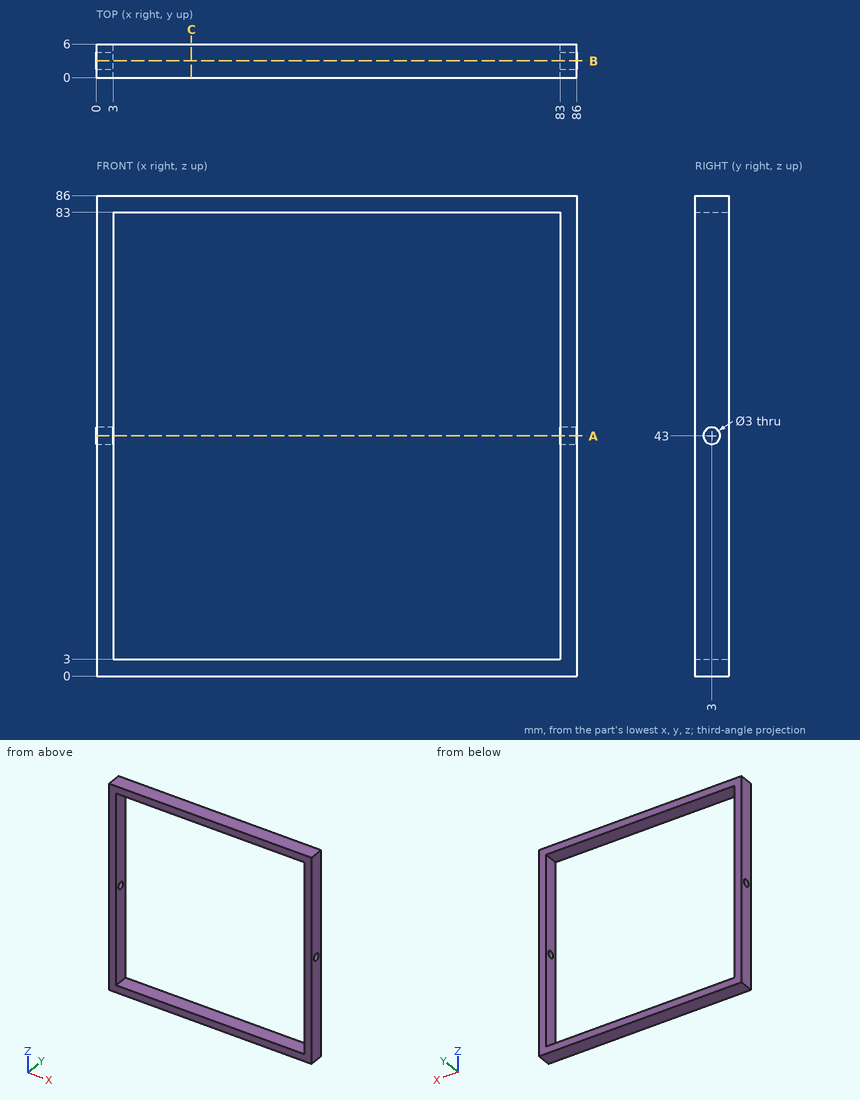
Can you work these out from the drawing? Everything is in mm from the part's minimum corner. Coordinates: 2 decimals unless noted, no trailing zeros. Loops run counter-clockwise (first coordinate to the right, second up) from the corner with the lowest first, then second, coordinate; pieces in that order, holes last. Notation, with made-up numbers: (54.25, 7) - (83.25, 7) arc R23 ccw to (83.25, 33) - close; hole circle Ø2 at (-11.75, -11.5). An arc over 180 degrees is marked (long way). Put each result on its own line as item: value. Start each with the question number.
Item 1: Suppose I cut it at C-C (x = 17). Please give me the cut outline in (y, z), and give its area (3 significant figures).
Item 2: If I drill on line 1 along Z through (x, y) = (78, 1.65); line 2 along Z through (x, y) = (1.5, 3), over which ranges is the centre line in solid material (lowest first)?
Item 3: Suppose I cut it at A-A (z = 43). Please give me the cut outline in (x, y), and give its area (3 significant figures).
Item 4: Suppose I cut it at B-B (y = 3). Please give me the cut outline in (x, z), and give its area (3 significant figures).
Item 5: For pin 1 (3 mm diameter, centred on x = 41, y = 3.5, fed in from -Z), with a flat end and sliding along its axis, tell me the tip position at first contact or that it passes through.
Here are the results:
1. outline: (0, 0) - (6, 0) - (6, 3) - (0, 3) - close; (0, 83) - (6, 83) - (6, 86) - (0, 86) - close
1. area: 36.0 mm²
2. line 1: 0 to 3, 83 to 86
2. line 2: 0 to 41.5, 44.5 to 86
3. outline: (0, 0) - (3, 0) - (3, 1.5) - (0, 1.5) - close; (0, 4.5) - (3, 4.5) - (3, 6) - (0, 6) - close; (83, 0) - (86, 0) - (86, 1.5) - (83, 1.5) - close; (83, 4.5) - (86, 4.5) - (86, 6) - (83, 6) - close
3. area: 18.0 mm²
4. outline: (0, 0) - (86, 0) - (86, 41.5) - (83, 41.5) - (83, 3) - (3, 3) - (3, 41.5) - (0, 41.5) - close; (0, 44.5) - (3, 44.5) - (3, 83) - (83, 83) - (83, 44.5) - (86, 44.5) - (86, 86) - (0, 86) - close
4. area: 978 mm²
5. pin 1: z = 0
